Check sheet for the modelled part. Datum: model origin and axes. Units: mm. A direction names the side the tool comes from. Round coordinates to 2 decimals unless told otherwise and drop trailing zeros. Write each loop counter-clockwise with the first axis right and the second up, starting at its lowest first coordinate (ties: lowest second). Pieces come first, ordered by that corner, then holes.
Item 1: Set-up check for faces 5 (the cylindrical face through (-50, -164.5, -473.9)), 6 (the flat face through (80, -209, -802)), 7 (the flat face through (1.4, -58.05, -60.47)): record each of +Z, -Z, +X, -X, +Y, -Y from which the full face is reachable in a straight line by a thin tool's end or side.
Item 2: Material ranges on line 1 along Y through (x, z) = (-79, -717); line 2 along Y through (x, z) = (-84.5, -396.5); line 3 along Z through (x, y) = (-53.5, -11.5), recorded low to high.
Item 3: Release check for a two-part mould opening along X. For faces 1 (the flat face through (1.4, -55.37, -66.34)), 2 (the flat face through (100, -155, -417)), 3 (the flat face through (-100, -155, -417)), 4 (the cylindrical face through (50.37, -164.53, -474.27)) record: pulls with the +X half, pulls with the -X half, needs draft (parallel to the pull), parting line crosses it, or undercut.
Item 4: Section check D-D, the plane z = -416.5. Record the cut outline in (x, y), plus the area to 3 significant figures.
Item 5: Section check C-C, the plane y = -140. Record the cut outline in (x, z).
Item 6: Depth check by flat-ended pin: pin 1 (4 mm diameter, centred on x = 13.5, y = -59.5, fed in from -Z). Enter the tip coordinate at first touch or a pass-through.
Item 7: Section check B-B, the plane z = -640.5. Record the cut outline in (x, y), plus the area to 3 significant figures.
Item 8: Section check A-A, the plane x = -13.5. Record the cut outline in (y, z).
from build123d import *

# Parameters (mm, degrees)
SM_BASE_FLANGE_1_DEPTH = 100
CUT_EXTRUDE_1_DEPTH    = 867.216543549
FILLET_1_R             = 25


# Sheet-metal steps are written as plain solids
with BuildPart() as part:
    # Sketch 1 → 基体-法兰1 (new, symmetric)
    with BuildSketch(Plane(origin=(0, 0, 0), x_dir=(0, 0, -1), z_dir=(1, 0, 0))):
        with BuildLine():
            Line((0, 0), (122.650248882, -117.744238927))
            ThreePointArc((122.650248882, -117.744238927), (125.224977196, -119.534385204), (128.227535984, -120.439089748))
            Line((128.227535984, -120.439089748), (838, -217))
            Line((838, -217), (838.808818708, -211.054765581))
            Line((838.808818708, -211.054765581), (129.036354692, -114.493855329))
            ThreePointArc((129.036354692, -114.493855329), (127.835331177, -114.131973511), (126.805439851, -113.415915001))
            Line((126.805439851, -113.415915001), (4.155190969, 4.328323926))
            Line((4.155190969, 4.328323926), (0, 0))
        make_face()
    extrude(amount=SM_BASE_FLANGE_1_DEPTH, both=True)

    # 草图4 → 切除-拉伸1 (cut, through all)
    with BuildSketch(Plane(origin=(0, -95.177553726, 12.94841895), x_dir=(1, 0, 0), z_dir=(0, 0.9908724031816991, -0.13480311796440184))):
        with BuildLine():
            Line((-80, 859.603350465), (-80, 788.103350465))
            ThreePointArc((-80, 788.103350465), (-77.008521077, 776.244809239), (-68.75, 767.224234104))
            ThreePointArc((-68.75, 767.224234104), (-60.491478923, 758.203658969), (-57.5, 746.345117743))
            Line((-57.5, 746.345117743), (-57.5, 484.603350465))
            Line((-57.5, 484.603350465), (57.5, 484.603350465))
            Line((57.5, 484.603350465), (57.5, 746.345117743))
            ThreePointArc((57.5, 746.345117743), (60.491478923, 758.203658969), (68.75, 767.224234104))
            ThreePointArc((68.75, 767.224234104), (77.008521077, 776.244809239), (80, 788.103350465))
            Line((80, 788.103350465), (80, 859.603350465))
            Line((80, 859.603350465), (-80, 859.603350465))
        make_face()
    extrude(amount=-CUT_EXTRUDE_1_DEPTH, mode=Mode.SUBTRACT)

    # 圆角1
    fillet_1_edges = [part.edges().sort_by_distance(p)[0] for p in [
        (57.5, -163.476213554, -466.827258161),
        (-57.5, -163.476213554, -466.827258161),
    ]]
    fillet(fillet_1_edges, radius=FILLET_1_R)


solid = part.part
Values found:
1. face 5: -Z, -Y
1. face 6: -Z, +Y, -Y
1. face 7: +Z, +X, -X, -Y
2. line 1: y = -200.54 to -194.48
2. line 2: y = -156.94 to -150.88
2. line 3: z = -20.64 to -11.98
3. face 1: needs draft
3. face 2: pulls with the +X half
3. face 3: pulls with the -X half
3. face 4: undercut
4. outline: (-100, -159.66) - (100, -159.66) - (100, -153.6) - (-100, -153.6) - close
4. area: 1,210 mm2
5. outline: (-100, -316.52) - (100, -316.52) - (100, -272.01) - (-100, -272.01) - close
6. pin 1: stops at z = -72.73
7. outline: (-100, -190.13) - (-57.5, -190.13) - (-57.5, -184.08) - (-100, -184.08) - close; (57.5, -190.13) - (100, -190.13) - (100, -184.08) - (57.5, -184.08) - close
7. area: 515 mm2
8. outline: (-166.45, -466.42) - (-160.5, -467.23) - (-114.49, -129.04) arc R4 cw to (-113.42, -126.81) - (4.33, -4.16) - (0, 0) - (-117.74, -122.65) arc R10 ccw to (-120.44, -128.23) - close
